Autodesk Fusion 360 part; units mm, degrees
sketch "Sketch1" plane through (0, 0, 0) normal (0, 0, 1) x (1, 0, 0)
  circle A0 centre (0, 0) radius 6.3
  circle A1 centre (0, 0) radius 7.6
  line L0 (0, 7.6) -> (0, -7.6) construction
  circle A2 centre (0, 0) radius 3.25
  line L1 (-3.25, 0) -> (-3.25, -3.35)
  line L2 (-3.25, -3.35) -> (3.25, -3.35)
  line L3 (3.25, 0) -> (3.25, -3.35)
  circle A3 centre (0, 0) radius 5
  dimension "d1" = 12.6
  dimension "d2" = 15.2
  dimension "d3" = 6.5
  dimension "d4" = 3.35
  dimension "d15" = 10
extrude "Extrude1" add sketch "Sketch1" along normal blind 0.4 contours A0 | A1
sketch "Sketch2" plane through (0, 0, 0.4) normal (0, 0, 1) x (-1, 0, 0)
  circle A0 centre (0, 0) radius 7.6
  circle A1 centre (0, 0) radius 6.125
  circle A2 centre (0, 0) radius 5.1
  line L0 (-10, -2.625) -> (10, -2.625)
  line L1 (10, -2.625) -> (10, 2.625)
  line L2 (10, 2.625) -> (-10, 2.625)
  line L3 (-10, 2.625) -> (-10, -2.625)
  line L4 (-10, -2.625) -> (10, 2.625) construction
  line L5 (10, -2.625) -> (-10, 2.625) construction
  circle A3 centre (0, 0) radius 5
  dimension "d7" = 12.25
  dimension "d8" = 10.2
  dimension "d9" = 5.25
  dimension "d10" = 20
extrude "Extrude2" add sketch "Sketch2" along normal blind 10 contours A1 A2 L0 L2 | A1 A2 L0 L2
fillet "Fillet1" radius 0.2 8 edges at (4.3726, -2.625, 5.4) (4.3726, 2.625, 5.4) (5.534, 2.625, 5.4) (5.534, -2.625, 5.4) (-4.3726, -2.625, 5.4) (-4.3726, 2.625, 5.4) (-5.534, 2.625, 5.4) (-5.534, -2.625, 5.4)
sketch "Sketch3" plane through (0, 0, 0) normal (0, 0, -1) x (1, 0, 0)
  circle A0 centre (0, 0) radius 5
  circle A1 centre (0, 0) radius 7.6
  line L0 (-7.25, 10) -> (7.25, 10)
  line L1 (7.25, 10) -> (7.25, -10)
  line L2 (7.25, -10) -> (-7.25, -10)
  line L3 (-7.25, -10) -> (-7.25, 10)
  line L4 (-7.25, 10) -> (7.25, -10) construction
  line L5 (7.25, 10) -> (-7.25, -10) construction
  dimension "d16" = 14.5
  dimension "d17" = 20
extrude "Extrude3" cut sketch "Sketch3" against normal blind 12 contours A1 L1 | A1 L3
equation "d4 = 6.6 mm - ( d3 / 2 )"
Model file for the job. Use its own axes, mm. A direction names the side the tool comes from. Coordinates: 2 decimals unless noted, no trailing zeros. Order: outer loops, then holes, each group sorted by start corner. A loop starts at its lowest first (then second) coordinate and runs counter-clockwise, first axis right, second up. Notation, with made-up numbers: (35.5, 43.25) - (75.5, 43.25) arc R26 cw to (75.5, 65.25) - close; hole circle Ø7 at (88.25, -7.5). An arc over 180 degrees is marked (long way). Return JSON: item names as keys, results as strings. Group by question number.
1) Probe line 1 (Y direction, x = 0, z = 0.2); line 2 (Z direction, x = -5.75, y = -4.75). List the from-to ranges inside material, lowest first. Write a range as from..to.
2) Saw through at C-C, the plane x = 0. Write the cut outline in (y, z), plus the area to 3 significant figures.
3) Saw through at D-D, the plane y = -3. Write the cut outline in (x, z), plus the area to 3 significant figures.
4) Saw through at B-B, the plane y = 0. Write the cut outline in (x, z) (3 decimals).
5) Flat gauge pins, fed straight in: P1, Ø2, axis at x = -2, y = 6, coming from the -Z side; P2, Ø0.6, axis at x = 5, z = 3, coming from the +Y side (3 decimals); P3, Ø5, axis at x = -0.5, y = 1.5, coming from the +Z side; P4, Ø0.8, axis at x = -5, z = 6, coming from the -Y side (3 decimals). Where does each tip first touch, or does it go through?
6) Mould opens along X. For faces 1 (the cylindrical face through (-5.1, 0, 5.3)), 2 (the cylindrical face through (-1.08, 4.88, 0.2)), 3 (the cylindrical face through (6.125, 0.036, 5.33)), 4 (the cylindrical face through (-0.1, 7.6, 0.2)) say: released by +X, released by -X, zero draft, split by the parting line, or undercut.
7) Tool access for faces 5 (the flat face through (-5.5, 0, 10.4)), 6 (the cylindrical face through (5.1, 0, 5.3)), 7 (the cylindrical face through (-6.125, -0.036, 5.33)): list every direction of +Z, -Z, +X, -X, +Y, -Y with a clear straight run to the whole face (end or side of a thin tool).
Values found:
{
 "1": {"line 1": "y = -7.6..-5, 5..7.6", "line 2": "z = 0..0.4"},
 "2": {"outline": "(-7.6, 0) - (-5, 0) - (-5, 0.4) - (-7.6, 0.4) - close; (5, 0) - (7.6, 0) - (7.6, 0.4) - (5, 0.4) - close", "area": "2.08 mm²"},
 "3": {"outline": "(-6.98, 0) - (-4, 0) - (-4, 0.4) - (-6.98, 0.4) - close; (4, 0) - (6.98, 0) - (6.98, 0.4) - (4, 0.4) - close", "area": "2.39 mm²"},
 "4": {"outline": "(-7.25, 0) - (-5, 0) - (-5, 0.4) - (-5.1, 0.4) - (-5.1, 10.4) - (-6.125, 10.4) - (-6.125, 0.4) - (-7.25, 0.4) - close; (5, 0) - (7.25, 0) - (7.25, 0.4) - (6.125, 0.4) - (6.125, 10.4) - (5.1, 10.4) - (5.1, 0.4) - (5, 0.4) - close"},
 "5": {"P1": "stops at z = 0", "P2": "stops at y = 2.625", "P3": "passes through", "P4": "stops at y = -2.625"},
 "6": {"face 1": "undercut", "face 2": "undercut", "face 3": "released by +X", "face 4": "split by the parting line"},
 "7": {"face 5": "+Z, +X, -X, +Y, -Y", "face 6": "+Z", "face 7": "+Z, -X"}
}
